Here's how the part is built. I have some questions about the finished solid (model axes, mm). A direction names the side the tool comes from. Coordinates: 2 decimals unless noted, no trailing zeros. Write each loop counter-clockwise with the first axis right and the second up, starting at its lowest first coordinate (ties: lowest second). Pieces come first, ordered by that corner, then holes.
Autodesk Inventor part; units mm, degrees
ref_plane "YZ Plane" through (0, 0, 0) normal (1, 0, 0) x (0, 1, 0)
ref_plane "XZ Plane" through (0, 0, 0) normal (0, 1, 0) x (-1, 0, 0)
ref_plane "XY Plane" through (0, 0, 0) normal (0, 0, 1) x (1, 0, 0)
sketch "Skizze2" plane through (0, 0, 0) normal (0, 1, 0) x (-1, 0, 0)
  line L0 (0, 0) -> (-20, 0)
  line L1 (-20, 0) -> (-20, 20)
  line L2 (-20, 20) -> (0, 20)
  line L3 (0, 20) -> (0, 0)
  dimension "d4" = 20
  dimension "d5" = 20
extrude "Extrusion2" add sketch "Skizze2" along normal blind 38
sketch "Skizze4" plane through (0, 0, 0) normal (-1, 0, 0) x (0, 0, 1)
  line L0 (20, 0) -> (0, 0)
  line L1 (0, 0) -> (20, 0)
  line L2 (20, 0) -> (20, 20)
  line L3 (20, 20) -> (0, 20)
  line L4 (0, 20) -> (0, 0)
  dimension "d8" = 20
  dimension "d9" = 20
extrude "Extrusion3" add sketch "Skizze4" along normal blind 17
fillet "Rundung1" radius 5 14 edges at (0, 20, 10) (-17, 20, 10) (-17, 0, 10) (20, 0, 10) (1.5, 0, 20) (20, 19, 20) (20, 19, 0) (0, 29, 20) (0, 29, 0) (-8.5, 20, 20) (-8.5, 20, 0) (-17, 10, 20) (-17, 10, 0) (1.5, 0, 0)
sketch "Skizze5" plane through (0, 0, 0) normal (0, -1, 0) x (1, 0, 0)
  line L0 (0, 5) -> (0, 15)
  line L1 (0, 10) -> (0, 20)
  line L2 (0, 10) -> (10, 10)
  point P0 (0, 0)
  dimension "d13" = 10
  dimension "d14" = 10
hole "Bohrung1" at (10, 0, 10) direction (0, 1, 0) diameter 8 end through all countersink diameter 10 countersink angle 90
properties part number "Stoper" material "PVC, hart"
1) I need wall thicknesses on probe 1 along Z at (x, y) = (10, 15); probe 2 along X at (y, z) = (15, 10); probe 3 along X at (y, z) = (34.5, 9.75). Which ranges of each line are inside material? Lowest first, please.
Values follow:
probe 1: z = 0 to 6, 14 to 20
probe 2: x = -17 to 6, 14 to 20
probe 3: x = 0 to 6.01, 13.99 to 20
2) Imagine slicing it at C-C on y = 32. Please give me the cut outline in (x, z), then the cut area to 3 significant figures.
Values follow:
outline: (0, 5) arc R5 ccw to (5, 0) - (15, 0) arc R5 ccw to (20, 5) - (20, 15) arc R5 ccw to (15, 20) - (5, 20) arc R5 ccw to (0, 15) - close; hole circle Ø8 at (10, 10)
area: 328 mm2
3) Imagine slicing it at B-B on z = 4. Please give me the cut outline in (x, y).
Values follow:
outline: (-16.9, 5) arc R4.9 ccw to (-12, 0.1) - (15, 0.1) arc R4.9 ccw to (19.9, 5) - (19.9, 38) - (0.1, 38) - (0.1, 25) arc R5.1 cw to (-5, 19.9) - (-12, 19.9) arc R4.9 ccw to (-16.9, 15) - close
4) On a 3-axis mill with a long thin cutter (end or side, diameter ignored), from which of +Z, -Z, +X, -X, +Y, -Y can I reach the whole of each face in a straight line? I mean faces 1 (the face through (0, 31, 10)), 2 (the face through (-16, 10, 2)), 3 (the face through (1, 32, 18)), 4 (the face through (1, 2, 1)), 5 (the face through (2, 32, 1)). Say none if no direction works.
Values follow:
face 1: +Z, -Z, -X, +Y
face 2: -Z, -X, +Y, -Y
face 3: +Z, -X, +Y
face 4: -Z, +X, -X, -Y
face 5: -Z, -X, +Y
5) Imagine slicing it at A-A on y = 10.5. Please give me the cut outline in (x, z).
Values follow:
outline: (-17, 5) arc R5 ccw to (-12, 0) - (15, 0) arc R5 ccw to (20, 5) - (20, 15) arc R5 ccw to (15, 20) - (-12, 20) arc R5 ccw to (-17, 15) - close; hole circle Ø8 at (10, 10)
6) Will these pins go through, and if not, where does the flat tip stop? pin 1 (8 mm diameter, centred on y = 32, z = 9, fed in from -X); pin 2 (5 mm diameter, centred on x = -13, z = 16, fed in from +Y); pin 3 (2 mm diameter, centred on x = -11, z = 17.5, fed in from -Y).
Values follow:
pin 1: stops at x = 0
pin 2: stops at y = 20
pin 3: stops at y = 0.23
